Geometry check sheet. Reference: drawing and pictorial views, mm from the part's lowest x, y, z. Coordinates: 2 decimals unless noted, no trailing zeros. Write each loop counter-clockwise with the first axis right and the second up, starting at its lowest first coordinate (ties: lowest second). Pieces come first, ordered by that corner, then holes. Notation, with made-up numbers: (42, 73.25) -> (96, 73.25) arc R19 cw to (96, 91.25) -> close; hole circle Ø4 at (55.5, 27). An arc over 180 degrees is marked (long way). Use a Markdown table: item, result.
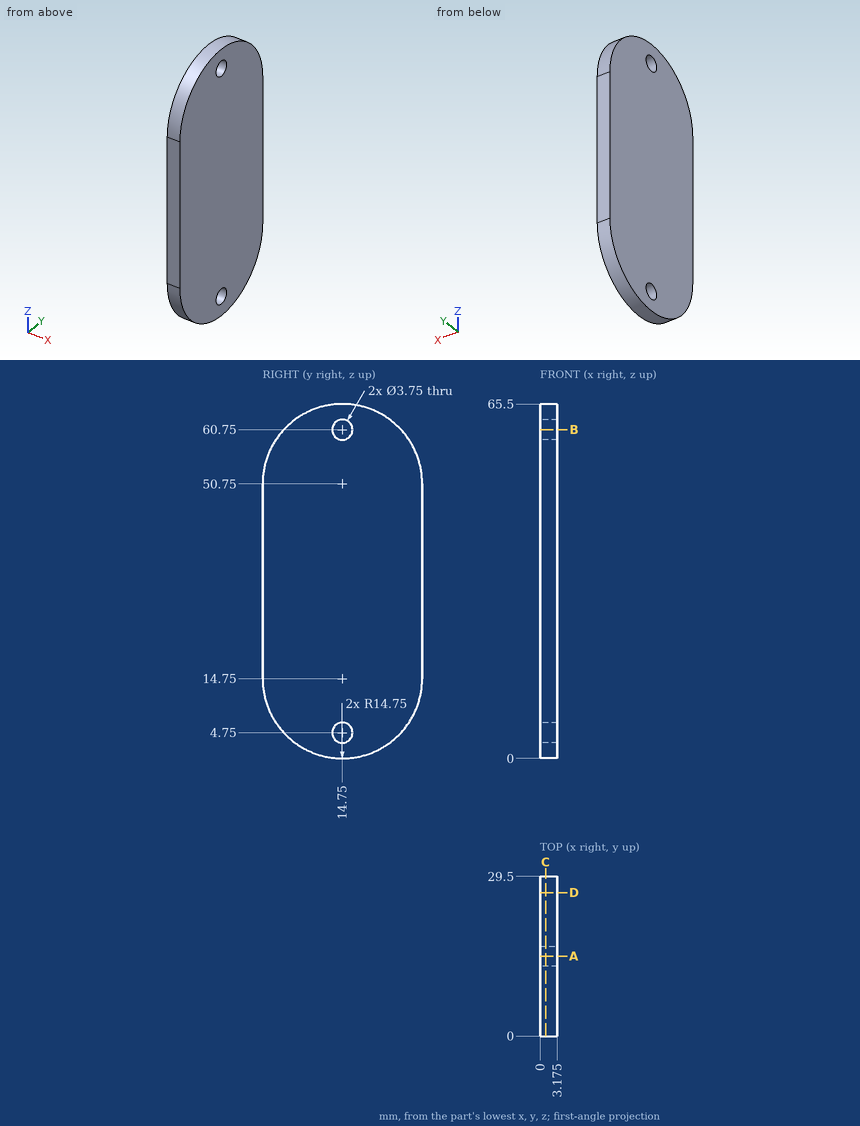
Item 1: Depth check by flat-ended pin: P1, Ø1, axis at x = 2, y = 5, coming from the -Z side; P2, Ø3.5, axis at y = 14.75, z = 60.75, coming from the +X side. Enter the tip coordinate at first touch or a pass-through.
Answer block:
| item | result |
|---|---|
| P1 | stops at z = 3.26 |
| P2 | passes through |
Item 2: Section check B-B on z = 60.75. Record the boundary of the cut face in (x, y) (3 decimals), then the cut area to 3 significant figures.
Answer block:
| item | result |
|---|---|
| outline | (0, 3.907) -> (3.175, 3.907) -> (3.175, 12.875) -> (0, 12.875) -> close; (0, 16.625) -> (3.175, 16.625) -> (3.175, 25.593) -> (0, 25.593) -> close |
| area | 56.9 mm^2 |
Item 3: Section check A-A on y = 14.75. Record the boundary of the cut face in (x, z) (3 decimals).
Answer block:
| item | result |
|---|---|
| outline | (0, 0) -> (3.175, 0) -> (3.175, 2.875) -> (0, 2.875) -> close; (0, 6.625) -> (3.175, 6.625) -> (3.175, 58.875) -> (0, 58.875) -> close; (0, 62.625) -> (3.175, 62.625) -> (3.175, 65.5) -> (0, 65.5) -> close |
Item 4: Section check C-C on x = 1. Record the boundary of the cut face in (y, z) (3 decimals).
Answer block:
| item | result |
|---|---|
| outline | (0, 14.75) arc R14.75 ccw to (29.5, 14.75) -> (29.5, 50.75) arc R14.75 ccw to (0, 50.75) -> close; hole circle Ø3.75 at (14.75, 4.75); hole circle Ø3.75 at (14.75, 60.75) |
Item 5: Section check D-D on y = 26.5. Record the boundary of the cut face in (x, z) (3 decimals).
Answer block:
| item | result |
|---|---|
| outline | (0, 5.834) -> (3.175, 5.834) -> (3.175, 59.666) -> (0, 59.666) -> close |
Item 6: Thickness scan on L1, parallel to Z at x = 1.2, y = 14.75 (3 decimals); L2, parallel to Y at x = 1.5, z = 60.75 (3 decimals); L3, parallel to Y at x = 0.2, z = 9. Record the ranges inside material, lowest first. Write a range as [from, to].
Answer block:
| item | result |
|---|---|
| L1 | z = [0, 2.875], [6.625, 58.875], [62.625, 65.5] |
| L2 | y = [3.907, 12.875], [16.625, 25.593] |
| L3 | y = [1.17, 28.33] |
